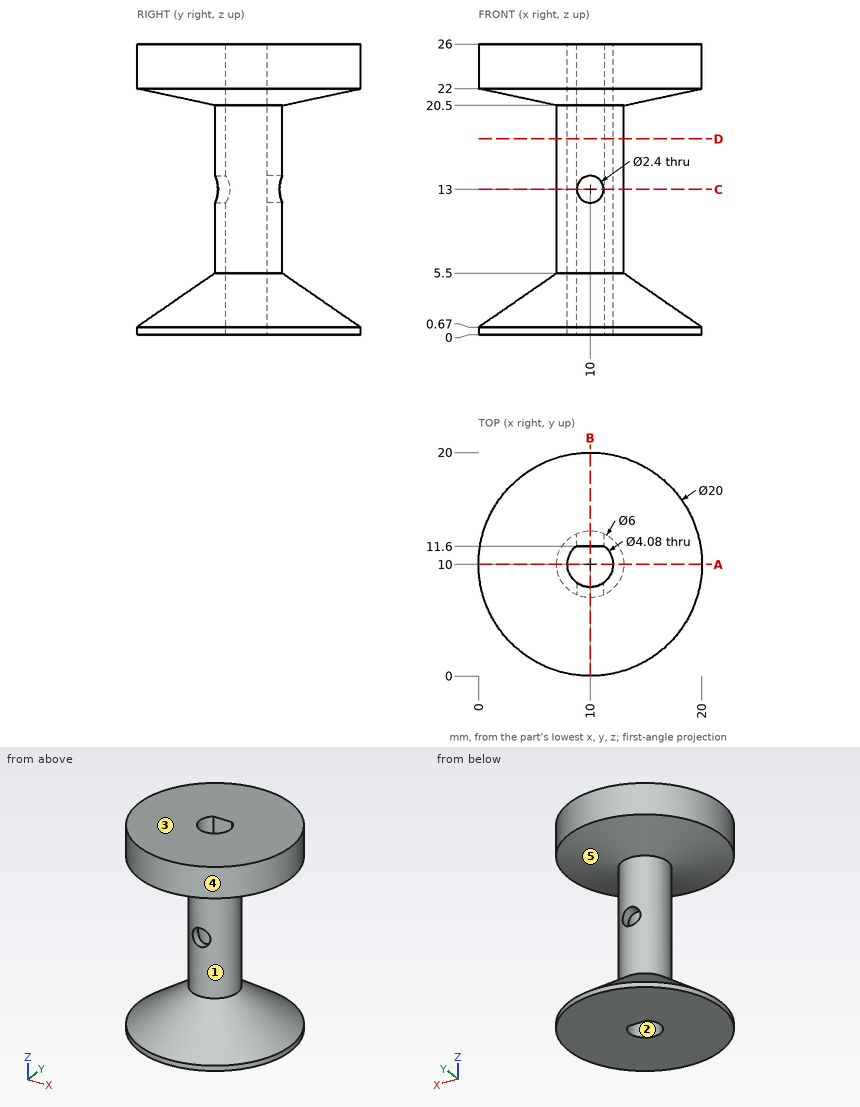
Verification items for this drawing (mm, ordinates from the low corner). A direction names the side the tool comes from. Give positions to 0.01 mm unless a question says otherwise; leave off trailing zeros. Loops run counter-clockwise (first coordinate to the right, second up) from the corner with the lowest first, then second, coordinate; pieces in that order, holes last. Notation, with made-up numbers: M -26,58.25 L -20,58.25 A17 cw -20,74.25 Z; hole C 7.5,43 d9. An arc over 180 degrees is marked long. Answer as a JSON object with one key per item and string values. Group by question number.
Q1. Cross-section at D-D on z = 17.5. Record the cut outline in (x, y), then the cut area to 3 significant figures.
Q2. Go/stop test with flat-tipped pins: P1, Ø2, axis at y = 11.5, z = 16.5, coming from the +X side; P2, Ø4, axis at y = 17.5, z = 23, coming from the -X side; P3, Ø2, axis at x = 10, z = 7.5, coming from the -Y side; P4, Ø8, axis at x = 11, y = 8.5, coming from the +Z side. Record where each tip stops, or that it passes through.
Q3. Cross-section at A-A on y = 10. Record the cut outline in (x, z), then the cut area to 3 significant figures.
Q4. Release check for a two-part mould opening along Y. For the marked faces 1, 2 and 3 record: released by +Y, released by -Y, zero draft, split by the parting line, or undercut.
Q5. Cross-section at C-C on z = 13. Record the cut outline in (x, y).
Q6. Cross-section at B-B on x = 10. Record the cut outline in (y, z), then the cut area to 3 significant figures.
Q7. Access from +Z, -Z, +X, -X, +Y, -Y to the whole of each face (thin tool, end or side, straight path). Record for the marked faces 4 and 5.
Q8. Material ranges on line 1 along Z through (x, y) = (10, 12); line 2 along Y through (x, z) = (10, 17.75); line 3 along Y through (x, z) = (11.5, 4.5), recorded low to high. Write a range as [from, to].
Evaluation:
{
 "1": {"outline": "C 10,10 d6; hole M 8.73,11.6 A2.04 ccw long 11.27,11.6 Z", "area": "16.0 mm2"},
 "2": {"P1": "stops at x = 12.96", "P2": "stops at x = 1.65", "P3": "stops at y = 7", "P4": "stops at z = 26"},
 "3": {"outline": "M 0,0 L 7.96,0 L 7.96,26 L 0,26 L 0,22 L 7,20.5 L 7,5.5 L 0,0.67 Z; M 12.04,0 L 20,0 L 20,0.67 L 13,5.5 L 13,20.5 L 20,22 L 20,26 L 12.04,26 Z", "area": "160 mm2"},
 "4": {"face 1": "split by the parting line", "face 2": "undercut", "face 3": "zero draft"},
 "5": {"outline": "M 8.73,11.6 L 8.8,11.6 L 8.8,12.75 A3 ccw 8.8,7.25 L 8.8,8.35 A2.04 cw Z; M 11.2,7.25 A3 ccw 11.2,12.75 L 11.2,11.6 L 11.27,11.6 A2.04 cw 11.2,8.35 Z"},
 "6": {"outline": "M 0,0 L 7.96,0 L 7.96,11.8 L 7,11.8 L 7,5.5 L 0,0.67 Z; M 0,22 L 7,20.5 L 7,14.2 L 7.96,14.2 L 7.96,26 L 0,26 Z; M 11.6,0 L 20,0 L 20,0.67 L 13,5.5 L 13,11.8 L 11.6,11.8 Z; M 11.6,14.2 L 13,14.2 L 13,20.5 L 20,22 L 20,26 L 11.6,26 Z", "area": "165 mm2"},
 "7": {"face 4": "+Z, -Z", "face 5": "none"},
 "8": {"line 1": "z = [0, 11.8], [14.2, 26]", "line 2": "y = [7, 7.96], [11.6, 13]", "line 3": "y = [5.81, 8.62], [11.38, 14.19]"}
}
